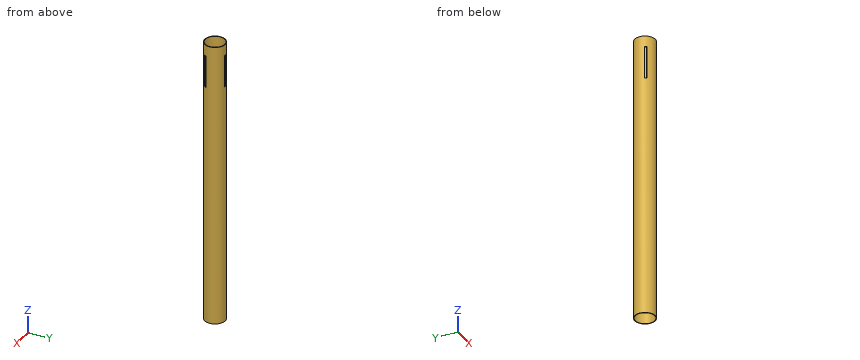
```python
from build123d import *

# Parameters (mm, degrees)
SKETCH1_R               = 19
SKETCH1_R_2             = 18
BOSS_EXTRUDE1_DEPTH     = 525
CUT_EXTRUDE1_REACH      = 528.716
CUT_EXTRUDE1_END_RADIUS = 18
SKETCH2_W               = 4
SKETCH2_H               = 60
CIRPATTERN1_COUNT       = 3


with BuildPart() as part:
    # Sketch1 → Boss-Extrude1 (new body)
    with BuildSketch(Plane.XY):
        Circle(SKETCH1_R)
        Circle(SKETCH1_R_2, mode=Mode.SUBTRACT)
    extrude(amount=BOSS_EXTRUDE1_DEPTH)

    # Cut-Extrude1: up to this cylinder (the profile starts outside it)
    cut_extrude1_end = Plane(origin=(0, 0, 475), z_dir=(0, 0, -1)) * Cylinder(CUT_EXTRUDE1_END_RADIUS, 1094.432, mode=Mode.PRIVATE)
    # Sketch2 → Cut-Extrude1 (cut, up to the surface)
    with BuildSketch(Plane(origin=(0, 19, 0), x_dir=(1, 0, 0), z_dir=(0, 1, 0)), mode=Mode.PRIVATE) as cut_extrude1_sk1:
        with Locations((0, -475)):
            Rectangle(SKETCH2_W, SKETCH2_H)
    cut_extrude1_tool1 = extrude(cut_extrude1_sk1.sketch, amount=-CUT_EXTRUDE1_REACH, mode=Mode.PRIVATE) - cut_extrude1_end
    cut_extrude1 = cut_extrude1_tool1.solids().sort_by_distance((0, 19, 475))[0]
    add(cut_extrude1, mode=Mode.SUBTRACT)

    # CirPattern1: Cut-Extrude1 ×3 about axis
    cirpattern1_axis = Axis((0, 0, 0), (0, 0, 1))
    for i in range(1, CIRPATTERN1_COUNT):
        add(cut_extrude1.rotate(cirpattern1_axis, i * 360 / CIRPATTERN1_COUNT), mode=Mode.SUBTRACT)


solid = part.part
```
The listing builds one solid part. Answer for the finished solid, in the listing's coordinates (mm). Coordinates: 2 decimals unless noted, no trailing zeros. Loops run counter-clockwise (first coordinate to the right, second up) from the corner with the lowest first, then second, coordinate; pieces in that order, holes last. Notation, with made-up numbers: (-37.75, 38.5) - (-11.75, 38.5) arc R24 ccw to (-11.75, 66.5) - close; hole circle Ø9 at (-5.75, 20.5). An arc over 180 degrees is marked (long way). Write item = value, one per line.
1) Section B-B (x = -8) is taken. Determine the outline of the cut face in (y, z), plus the area to 3 significant figures.
Responses:
outline = (-17.23, 0) - (-16.12, 0) - (-16.12, 525) - (-17.23, 525) - close; (16.12, 0) - (17.23, 0) - (17.23, 525) - (16.12, 525) - close
area = 1,160 mm^2
2) Find the intervals of material crossed by line 1 along Y through (x, z) = (0, 190); line 2 along Y through (x, z) = (-1.5, 334.5); line 3 along X through (y, z) = (-15.5, 226), in increasing order.
Responses:
line_1 = -19 to -18, 18 to 19
line_2 = -18.94 to -17.94, 17.94 to 18.94
line_3 = -10.99 to -9.15, 9.15 to 10.99
3) Section C-C (z = 437) is taken. Determine the outline of the cut face in (x, y), plus the area to 3 significant figures.
Responses:
outline = circle Ø38 at (0, 0); hole circle Ø36 at (0, 0)
area = 116 mm^2
4) Each of these flat-tipped pins is pushed along its axis until it touches: P1, Ø4, axis at y = -9.5, z = 66, coming from the +X side; P2, Ø8, axis at y = -4.5, z = 426, coming from the +X side; P3, Ø2.5, axis at x = 15.5, y = -8.5, coming from the -Z side; P4, Ø1, axis at y = 1.5, z = 199.5, coming from the -X side. Where does it stop, or does it pass through?
Responses:
P1 = 17.46
P2 = 18.99
P3 = 0
P4 = -18.97
5) Section A-A (y = 0) is taken. Determine the outline of the cut face in (x, z), plus the area to 3 significant figures.
Responses:
outline = (-19, 0) - (-18, 0) - (-18, 525) - (-19, 525) - close; (18, 0) - (19, 0) - (19, 525) - (18, 525) - close
area = 1,050 mm^2
